Can you work these out from the model? Positions are in its coordinate system, mm. A direction names the side the tool comes from. Round coordinates to 2 decimals unless told otherwise and drop trailing zeros. Order: outer loops, then holes, each group sorted by start corner. A loop starts at its lowest first (then second) coordinate and runs counter-clockwise, first axis right, second up. Notation, with made-up numbers: (84, -4.75) -> (100, -4.75) arc R18 cw to (100, 27.25) -> close; hole circle Ø10 at (17.5, -32). An arc over 180 degrees is marked (long way). Use a Markdown table: item, result. Add a question column.
Q1. I need wall thicknesses on line 1 along Z through (x, y) = (1.5, 30); line 2 along Y through (x, z) = (4.5, 9.5); line 3 along X through (y, z) = (49, -0.75). Which ranges of each line are inside material? Lowest first, please. Write a range as [from, to].
Q2. If we section it at B-B on x = 4.5: List the corners of the cut face in (y, z) for me.
Q3. If we section it at D-D on z = 2.5: List the corners of the cut face in (x, y) for me, plus the area to 3 significant figures.
Q4. For faces 5 (the face through (3, 4, 4)), 6 (the face through (16.461, 1.014, -4.993)), 7 (the face through (1, 35, 10.5)), which set-ups out of +Z, -Z, +X, -X, +Y, -Y let a thin tool reach every point of the face, with its end or its side?
Q5. I'm going to push flat-ended pins straight in: pin 1 Ø2.5 at (x, y) = (5, 4) entering from +Z; pin 2 Ø0.6 at (x, y) = (0.5, 24.5) entering from +Z; pin 3 Ø4 at (x, y) = (5.5, 6.5) entering from -Z. Where does each tip first touch, or does it pass through?
Q6. If we section it at C-C on x = 18: List the corners of the cut face in (y, z) for me.
Q7. If we section it at A-A on y = 30: List the corners of the cut face in (x, z) for me.
Q8. We'd pull the mould along Z, two halves only. Please class faces 1 (the face through (3, 4, 8)), 2 (the face through (3, 56, -8)), 3 (the face through (4.5, 5.5, -6)), 4 (the face through (16.68, 1.01, 5.11)): +Z half, -Z half, draft (parallel to the pull), parting line (faces both ways), or undercut.
```python
from build123d import *

# Parameters (mm, degrees)
BOSS_EXTRUDE2_DEPTH = 12.5
CUT_EXTRUDE1_DEPTH  = 67.191011474
FILLET1_R           = 1
SKETCH7_R           = 1.5
CUT_EXTRUDE2_DEPTH  = 10
BOSS_EXTRUDE8_DEPTH = 8
CUT_EXTRUDE4_DEPTH  = 4
SKETCH15_W          = 2
SKETCH15_H          = 4
CUT_EXTRUDE5_DEPTH  = 2


with BuildPart() as part:
    # Sketch1 → Boss-Extrude2 (new, symmetric)
    with BuildSketch(Plane.XY):
        Polygon((0, 0), (0, 60), (25, 60), (25, 58), (2, 58), (2, 2), (25, 2), (25, 0), align=None)
    extrude(amount=BOSS_EXTRUDE2_DEPTH, both=True)

    # Sketch6 → Cut-Extrude1 (cut, through all)
    with BuildSketch(Plane(origin=(0, 60, 0), x_dir=(1, 0, 0), z_dir=(0, 1, 0))):
        Polygon((7, 0), (25, 9.5), (25, -9.5), align=None)
    extrude(amount=-CUT_EXTRUDE1_DEPTH, mode=Mode.SUBTRACT)

    # Fillet1
    fillet1_edges = [part.edges().sort_by_distance(p)[0] for p in [
        (25, 1, 9.5),
        (25, 59, 9.5),
        (7, 1, 0),
        (7, 59, 0),
        (25, 1, -9.5),
        (25, 59, -9.5),
    ]]
    fillet(fillet1_edges, radius=FILLET1_R)

    # Sketch7 → Cut-Extrude2 (cut)
    with BuildSketch(Plane(origin=(2, 0, 0), x_dir=(0, 0, -1), z_dir=(1, 0, 0))):
        with Locations(Location((0.18959721, 30, 0), (0, 0, 90))):
            Circle(SKETCH7_R)
        with Locations(Location((10, 30, 0), (0, 0, 90))):
            Circle(SKETCH7_R)
    extrude(amount=-CUT_EXTRUDE2_DEPTH, mode=Mode.SUBTRACT)

    # Sketch13 → Boss-Extrude8 (add, symmetric)
    with BuildSketch(Plane.XY):
        Polygon((2, 58), (7, 58), (2, 51), align=None)
        Polygon((7, 2), (2, 2), (2, 9), align=None)
    extrude(amount=BOSS_EXTRUDE8_DEPTH, both=True)

    # Sketch14 → Cut-Extrude4 (cut, symmetric)
    with BuildSketch(Plane.XY):
        Polygon((2, 2), (2, 9), (7, 2), align=None)
        Polygon((2, 58), (7, 58), (2, 51), align=None)
    extrude(amount=CUT_EXTRUDE4_DEPTH, both=True, mode=Mode.SUBTRACT)

    # Sketch15 → Cut-Extrude5 (cut)
    with BuildSketch(Plane(origin=(2, 0, 0), x_dir=(0, 0, -1), z_dir=(1, 0, 0))):
        with Locations((-11.5, 35.5)):
            Rectangle(SKETCH15_W, SKETCH15_H)
        with Locations((-11.5, 24.5)):
            Rectangle(SKETCH15_W, SKETCH15_H)
    extrude(amount=-CUT_EXTRUDE5_DEPTH, mode=Mode.SUBTRACT)


solid = part.part
```
Answer below:
| question | item | result |
|---|---|---|
| 1 | line 1 | [-12.5, -11.5], [-8.5, -1.69], [1.31, 12.5] |
| 1 | line 2 | [0, 2], [58, 60] |
| 1 | line 3 | [0, 2] |
| 2 | outline | (0, -12.5) -> (2, -12.5) -> (2, -8) -> (5.5, -8) -> (5.5, -4) -> (2, -4) -> (2, 4) -> (5.5, 4) -> (5.5, 8) -> (2, 8) -> (2, 12.5) -> (0, 12.5) -> close; (54.5, -8) -> (58, -8) -> (58, -12.5) -> (60, -12.5) -> (60, 12.5) -> (58, 12.5) -> (58, 8) -> (54.5, 8) -> (54.5, 4) -> (58, 4) -> (58, -4) -> (54.5, -4) -> close |
| 3 | outline | (0, 0) -> (11.74, 0) -> (11.74, 2) -> (2, 2) -> (2, 58) -> (11.74, 58) -> (11.74, 60) -> (0, 60) -> close |
| 3 | area | 159 mm² |
| 4 | face 5 | +X |
| 4 | face 6 | +X, +Y, -Y |
| 4 | face 7 | +Z, +X, -X |
| 5 | pin 1 | z = 8 |
| 5 | pin 2 | z = 10.5 |
| 5 | pin 3 | z = -8 |
| 6 | outline | (0, -12.5) -> (2, -12.5) -> (2, -5.81) -> (0, -5.81) -> close; (0, 5.81) -> (2, 5.81) -> (2, 12.5) -> (0, 12.5) -> close; (58, -12.5) -> (60, -12.5) -> (60, -5.81) -> (58, -5.81) -> close; (58, 5.81) -> (60, 5.81) -> (60, 12.5) -> (58, 12.5) -> close |
| 7 | outline | (0, -12.5) -> (2, -12.5) -> (2, -11.5) -> (0, -11.5) -> close; (0, -8.5) -> (2, -8.5) -> (2, -1.69) -> (0, -1.69) -> close; (0, 1.31) -> (2, 1.31) -> (2, 12.5) -> (0, 12.5) -> close |
| 8 | face 1 | +Z half |
| 8 | face 2 | -Z half |
| 8 | face 3 | draft |
| 8 | face 4 | undercut |
